Part model, mm, in its own coordinate system. A direction names the side the tool comes from. Coordinates: 2 decimals unless noted, no trailing zeros. Order: outer loops, then holes, each group sorted by start corner. A loop starts at its lowest first (then second) coordinate and runs counter-clockwise, first axis right, second up.
Autodesk Inventor part; units mm, degrees
ref_plane "YZ Plane" through (0, 0, 0) normal (1, 0, 0) x (0, 1, 0)
ref_plane "XZ Plane" through (0, 0, 0) normal (0, 1, 0) x (-1, 0, 0)
ref_plane "XY Plane" through (0, 0, 0) normal (0, 0, 1) x (1, 0, 0)
sketch "Sketch1" plane through (0, 0, 0) normal (0, 1, 0) x (-1, 0, 0)
  arc A0 (9, -28.6182) -> (-9, -28.6182) centre (0, 0) ccw
  arc A1 (-5, 49.7494) -> (-5, -49.7494) centre (0, 0) ccw construction
  line L0 (0, 0) -> (-200, 0) construction
  arc A2 (-170, 0) -> (-200, 30) centre (-200, 0) ccw construction
  line L1 (-200, 30) -> (-200, -30) construction
  line L2 (-5, -49.7494) -> (-203, -29.8496)
  line L3 (-5, 49.7494) -> (-203, 29.8496)
  arc A3 (-5, -49.7494) -> (-5, 49.7494) centre (0, 0) ccw
  arc A4 (-200, -30) -> (-170, 0) centre (-200, 0) ccw construction
  arc A5 (-200, 30) -> (-200, -30) centre (-200, 0) ccw
  line L4 (0, 0) -> (0, -30) construction
  line L5 (9, -23) -> (-9, -23) construction
  line L6 (9, -23) -> (9, -28.6182) construction
  line L7 (-9, -23) -> (-9, -28.6182) construction
  line L8 (9, -28.6182) -> (9, -34)
  line L9 (-9, -28.6182) -> (-9, -34)
  line L10 (9, -34) -> (-9, -34)
  arc A6 (0, -30) -> (9, -28.6182) centre (0, 0) ccw construction
  arc A7 (-9, -28.6182) -> (0, -30) centre (0, 0) ccw construction
  dimension "d0" = 60
  dimension "d1" = 100
  dimension "d2" = 200
  dimension "d3" = 60
  dimension "d5" = 18
  dimension "d6" = 7
  dimension "d7" = 4
extrude "Extrusion1" add sketch "Sketch1" along normal blind 51.2
sketch "Sketch2" plane through (0, 51.2, 0) normal (0, 1, 0) x (1, 0, 0)
  arc A0 (203, -29.8496) -> (203, 29.8496) centre (200, 0) ccw
  circle A1 centre (200, 0) radius 12.7
  point P0 (0, 0)
  dimension "d10" = 25.4
extrude "Extrusion4" cut sketch "Sketch2" against normal through all
sketch "Sketch4" plane through (-9, 0, -34) normal (0, 0, 1) x (1, 0, 0)
  line L0 (0, 0) -> (18, 0)
  line L1 (18, 0) -> (18, 51.2)
  line L2 (0, 51.2) -> (18, 51.2)
  line L3 (0, 0) -> (0, 51.2)
  line L4 (9, 51.2) -> (9, 0) construction
  line L5 (0, 0) -> (0, 51.2) construction
  line L6 (0, 25.6) -> (18, 25.6) construction
  circle A0 centre (9, 25.6) radius 7.9375
  dimension "d24" = 15.875
extrude "Extrusion5" cut sketch "Sketch4" against normal through all contours A0
thread "Thread3"
properties part number "placa manivela" material "Steel, Carbon"
Q1. Cut at D-D on y = 5. Write the cut outline in (x, z).
Results list:
outline: (5, -49.75) - (203, -29.85) arc R30 ccw to (203, 29.85) - (5, 49.75) arc R50 ccw (long way) to start; hole (-9, -34) - (9, -34) - (9, -28.62) arc R30 ccw (long way) to (-9, -28.62) - close; hole circle Ø25.4 at (200, 0)
Q2. Wall check: line 1 along Y through (x, z) = (0, -42); line 2 along X through (y, z) = (23.5, 5); line 3 along X through (y, z) = (49.5, 3). Give the ranges that are in metal, low to high.
Results list:
line 1: y = 0 to 17.66, 33.54 to 51.2
line 2: x = -49.75 to -29.58, 29.58 to 188.33, 211.67 to 229.58
line 3: x = -49.91 to -29.85, 29.85 to 187.66, 212.34 to 229.85
Q3. Cut at B-B on z = 0. Write the cut outline in (x, y).
Results list:
outline: (-50, 0) - (-30, 0) - (-30, 51.2) - (-50, 51.2) - close; (30, 0) - (187.3, 0) - (187.3, 51.2) - (30, 51.2) - close; (212.7, 0) - (230, 0) - (230, 51.2) - (212.7, 51.2) - close
Q4. Pin check, flat tips, straight feed: pin 1 Ø8 at (x, z) = (69.5, 11.5) entering from -Y; pin 2 Ø8 at (x, y) = (114.5, 29.5) entering from -Z; pin 3 Ø14.5 at (x, y) = (0, 25.6) entering from -Z; pin 4 Ø5 at (x, y) = (142, 12.5) entering from +Z. Stop position of each tip, or through.
Results list:
pin 1: stops at y = 0
pin 2: stops at z = -39.15
pin 3: stops at z = 29.11
pin 4: stops at z = 36.23
Q5. Which spindle directions (+Z, -Z, +X, -X, +Y, -Y) get a long thin tool onto all of the face, cutting with end or side? Do faces 1 (the face through (-8.1, 25.2, -34)), 2 (the face through (92, 0, 1)). Say none if no direction does.
Results list:
face 1: +Y, -Y
face 2: +Z, -Z, +X, -X, -Y
Q6. Cut at C-C on x = 192. Write the cut outline in (y, z).
Results list:
outline: (0, -30.96) - (51.2, -30.96) - (51.2, -9.86) - (0, -9.86) - close; (0, 9.86) - (51.2, 9.86) - (51.2, 30.96) - (0, 30.96) - close
Q7. Mould opens along Z. For faces 3 (the face through (-1.72, 17.85, -41.89)), 4 (the face through (212.114, 25.958, -3.815)), 5 (the face through (1.191, 25.242, 29.976)), 6 (the face through (-49.986, 25.242, 1.17)) say: pulls with the +Z half, pulls with the -Z half, needs draft (parallel to the pull), parting line crosses it, or undercut.
Results list:
face 3: needs draft
face 4: undercut
face 5: undercut
face 6: parting line crosses it
Q8. Cut at A-A on x = 0. Write the cut outline in (y, z), and give its area (3 significant figures).
Results list:
outline: (0, -50) - (17.66, -50) - (17.66, -34) - (0, -34) - close; (0, 30) - (51.2, 30) - (51.2, 50) - (0, 50) - close; (33.54, -50) - (51.2, -50) - (51.2, -34) - (33.54, -34) - close
area: 1,590 mm2
